Geometry check sheet. Reference: the model listing, model coordinates, mm. A direction names the side the tool comes from. Round coordinates to 2 decimals unless told otherwise and drop trailing zeros. Write each loop counter-clockwise with the first axis right and the second up, starting at its lowest first coordinate (ties: lowest second). Pieces come first, ordered by that corner, then holes. Notation, with made-up numbers: M -15.5,-13 L 3.5,-13 A28 cw 3.5,22 Z; hole C 36.5,42 d1. An arc over 180 degrees is marked long. One line per item, written item: value. Start each with the question number.
1. Section check D-D (z = 9.5). Record the boundary of the cut face in (x, y), and give its area (3 significant figures).
2. Scan lines: probe 1 along X at (y, z) = (5, -0.5); probe 2 along Z at (x, y) = (0, 78); probe 3 along X at (y, z) = (79, -12). Record each from-to range of solid material in increasing order. Write a range as [from, to].
3. Section check C-C (y = 27). Record the boundary of the cut face in (x, z), and give its area (3 significant figures).
4. Depth check by flat-ended pin: P1, Ø0.9, axis at x = 0, z = -25.5, coming from the +Y side; P2, Ø1, axis at y = 13, z = -16.5, coming from the +X side; P3, Ø8, axis at y = 8.5, z = -26, coming from the -X side. Enter the tip coordinate at first touch or a pass-through.
5. Section check A-A (x = 0). Record the boundary of the cut face in (y, z).
6. Section check B-B (z = -9). Record the boundary of the cut face in (x, y), and give its area (3 significant figures).
7. Access from +Z, -Z, +X, -X, +Y, -Y to the whole of each face (thin tool, end or side, straight path). Record for faces 3 (the cylindrical face through (8.47, 3.451, -13.697)), 4 (the cylindrical face through (23.082, 77.549, -11.906)), 5 (the flat face through (0, 0, 0)).
8. Release check for a two-part mould opening along Z. For faces 1 (the flat face through (-22, 74, -13)), 2 (the flat face through (0, 81, 0)) record: pulls with the +Z half, pulls with the -Z half, needs draft (parallel to the pull), parting line crosses it, or undercut.
from build123d import *

# Parameters (mm, degrees)
CROQUIS1_R              = 35.5
SALIENTE_EXTRUIR1_DEPTH = 81
CROQUIS2_R              = 26
CROQUIS2_R_2            = 20
CORTAR_EXTRUIR1_DEPTH   = 7
CROQUIS3_R              = 1.6
CORTAR_EXTRUIR2_DEPTH   = 7
CROQUIS4_R              = 1.55
CORTAR_EXTRUIR3_DEPTH   = 7


with BuildPart() as part:
    # Croquis1 → Saliente-Extruir1 (new body)
    with BuildSketch(Plane(origin=(0, 0, 0), x_dir=(1, 0, 0), z_dir=(0, 1, 0))):
        Circle(CROQUIS1_R)
    extrude(amount=SALIENTE_EXTRUIR1_DEPTH)

    # Croquis2 → Cortar-Extruir1 (cut)
    with BuildSketch(Plane.XZ):
        Circle(CROQUIS2_R)
        Circle(CROQUIS2_R_2, mode=Mode.SUBTRACT)
    extrude(amount=-CORTAR_EXTRUIR1_DEPTH, mode=Mode.SUBTRACT)

    # Croquis3 → Cortar-Extruir2 (cut)
    with BuildSketch(Plane.XZ):
        with Locations((0, 15)):
            Circle(CROQUIS3_R)
        with Locations((14.265847744, 4.635254916)):
            Circle(CROQUIS3_R)
        with Locations((8.816778784, -12.135254916)):
            Circle(CROQUIS3_R)
        with Locations((-8.816778784, -12.135254916)):
            Circle(CROQUIS3_R)
        with Locations((-14.265847744, 4.635254916)):
            Circle(CROQUIS3_R)
    extrude(amount=-CORTAR_EXTRUIR2_DEPTH, mode=Mode.SUBTRACT)

    # Croquis4 → Cortar-Extruir3 (cut)
    with BuildSketch(Plane(origin=(0, 81, 0), x_dir=(1, 0, 0), z_dir=(0, 1, 0))):
        with Locations((0, 25)):
            Circle(CROQUIS4_R)
        with Locations((21.650635095, 12.5)):
            Circle(CROQUIS4_R)
        with Locations((21.650635095, -12.5)):
            Circle(CROQUIS4_R)
        with Locations((0, -25)):
            Circle(CROQUIS4_R)
        with Locations((-21.650635095, -12.5)):
            Circle(CROQUIS4_R)
        with Locations((-21.650635095, 12.5)):
            Circle(CROQUIS4_R)
    extrude(amount=-CORTAR_EXTRUIR3_DEPTH, mode=Mode.SUBTRACT)


solid = part.part
Result sheet:
1. outline: M -34.21,0 L -24.2,0 L -24.2,7 L -17.6,7 L -17.6,0 L 17.6,0 L 17.6,7 L 24.2,7 L 24.2,0 L 34.21,0 L 34.21,81 L -34.21,81 Z
1. area: 5,450 mm2
2. probe 1: x = [-35.5, -26], [-19.99, 19.99], [26, 35.5]
2. probe 2: z = [-35.5, -26.55], [-23.45, 23.45], [26.55, 35.5]
2. probe 3: x = [-33.41, -23.12], [-20.18, 20.18], [23.12, 33.41]
3. outline: C 0,0 d71
3. area: 3,960 mm2
4. P1: stops at y = 74
4. P2: stops at x = 31.69
4. P3: stops at x = -27.86
5. outline: M 0,-35.5 L 81,-35.5 L 81,-26.55 L 74,-26.55 L 74,-23.45 L 81,-23.45 L 81,23.45 L 74,23.45 L 74,26.55 L 81,26.55 L 81,35.5 L 0,35.5 L 0,26 L 7,26 L 7,20 L 0,20 L 0,16.6 L 7,16.6 L 7,13.4 L 0,13.4 L 0,-20 L 7,-20 L 7,-26 L 0,-26 Z
6. outline: M -34.34,0 L -24.39,0 L -24.39,7 L -17.86,7 L -17.86,0 L 17.86,0 L 17.86,7 L 24.39,7 L 24.39,0 L 34.34,0 L 34.34,81 L -34.34,81 Z
6. area: 5,470 mm2
7. face 3: -Y
7. face 4: +Y
7. face 5: +Z, -Z, +X, -X, -Y
8. face 1: undercut
8. face 2: needs draft
